Build history of the part. All positions in model axes, mm. A direction names the side the tool comes from. Round coordinates to 2 decimals unless told otherwise and drop trailing zeros. Write each loop counter-clockwise with the first axis right and the second up, starting at its lowest first coordinate (ties: lowest second). Pieces come first, ordered by that corner, then holes. Notation, with made-up numbers: M -21,48.25 L 4,48.25 A27 ccw 4,87.25 Z; hole C 77.25,80.25 d8. An arc over 180 degrees is marked long. Write item = value, one per line.
from build123d import *

# Parameters (mm, degrees)
BOSS_EXTRUDE1_DEPTH = 15
SKETCH2_R           = 2.1
CUT_EXTRUDE1_DEPTH  = 66.331515512
FILLET2_R           = 1.905


with BuildPart() as part:
    # Sketch1 → Boss-Extrude1 (new body)
    with BuildSketch(Plane(origin=(0, 0, 0), x_dir=(0, 0, -1), z_dir=(1, 0, 0))):
        with BuildLine():
            Line((-6.5, 0), (-10.31, 0))
            Line((-10.31, 0), (-10.31, 25.4))
            add(Edge.make_bspline(
                [(-10.31, 25.4), (-3.368064257, 40.422360056), (-3, 57.15)],
                knots=[0, 0, 0, 1, 1, 1], degree=2))
            ThreePointArc((-3, 57.15), (0, 60.15), (3, 57.15))
            add(Edge.make_bspline(
                [(10.31, 25.4), (3.368064257, 40.422360056), (3, 57.15)],
                knots=[0, 0, 0, 1, 1, 1], degree=2))
            Line((10.31, 25.4), (10.31, 0))
            Line((10.31, 0), (6.5, 0))
            Line((6.5, 0), (6.5, 25.4))
            Line((6.5, 25.4), (-6.5, 25.4))
            Line((-6.5, 25.4), (-6.5, 0))
        make_face()
    extrude(amount=BOSS_EXTRUDE1_DEPTH)

    # Sketch2 → Cut-Extrude1 (cut, through all)
    with BuildSketch(Plane(origin=(0, 0, -10.31), x_dir=(-1, 0, 0), z_dir=(0, 0, -1))):
        with Locations((-7.5, 7)):
            Circle(SKETCH2_R)
        with Locations((-7.5, 17)):
            Circle(SKETCH2_R)
    extrude(amount=-CUT_EXTRUDE1_DEPTH, mode=Mode.SUBTRACT)

    # Fillet2
    fillet2_edges = [part.edges().sort_by_distance(p)[0] for p in [
        (7.5, 25.4, -10.31),
        (7.5, 0, -10.31),
        (7.5, 0, -6.5),
        (7.5, 0, 6.5),
        (7.5, 0, 10.31),
        (7.5, 25.4, -6.5),
        (7.5, 25.4, 6.5),
        (7.5, 25.4, 10.31),
    ]]
    fillet(fillet2_edges, radius=FILLET2_R - 0.0001)  # a hair under: the kernel refuses the full size


solid = part.part
1. Band-saw the part on B-B (x = 7.5). Count the separate pieces of the cut face and the enclosed holes in it, plus the area to 3 significant figures.
Responses:
separate_pieces = 5
enclosed_holes = 0
area = 491 mm²
2. Mould opens along Y. For faces 3 (the face through (7.773, 9.082, -8.432)), 4 (the face through (7, 13, 6.5)), 5 (the face through (7.4, 60.15, 0.07)), 6 (the face through (7, 25.4, 0)) say: pulls with the +Y half, pulls with the -Y half, needs draft (parallel to the pull), parting line crosses it, or undercut.
Responses:
face_3 = undercut
face_4 = needs draft
face_5 = pulls with the +Y half
face_6 = pulls with the -Y half
3. Band-saw the part on A-A (y = 17). List the corners of the cut face in (x, z), plus the area to 3 significant figures.
Responses:
outline = M 0,-10.31 L 5.4,-10.31 L 5.4,-6.5 L 0,-6.5 Z; M 0,6.5 L 5.4,6.5 L 5.4,10.31 L 0,10.31 Z; M 9.6,-10.31 L 15,-10.31 L 15,-6.5 L 9.6,-6.5 Z; M 9.6,6.5 L 15,6.5 L 15,10.31 L 9.6,10.31 Z
area = 82.3 mm²
4. Flat gauge pins, fed straight in: pin 1 (1 mm diameter, centred on x = 4.5, y = 33, fed in from -Z); pin 2 (3 mm diameter, centred on x = 9.5, y = 34, fed in from +Z); pin 3 (7.5 mm diameter, centred on x = 9, z = 1.5, fed in from -Y). Where does each tip first touch, or does it go through?
Responses:
pin_1 = -7.43
pin_2 = 7.43
pin_3 = 25.28
5. Band-saw the part on C-C (z = 0). List the corners of the cut face in (x, y).
Responses:
outline = M 0,25.4 L 15,25.4 L 15,60.15 L 0,60.15 Z
6. Tool access for faces 1 (the face through (7.605, 24.827, 5.957)), 2 (the face through (7, 13, 10.31)): list every direction of +Z, -Z, +X, -X, +Y, -Y with a clear straight run to the whole face (end or side of a thin tool).
Responses:
face_1 = +X, -X, -Y
face_2 = +Z, +X, -X, +Y, -Y
7. Probe probe 1 along Z at (x, y) = (11, 18.5); probe 2 along X at (y, z) = (16, -9); probe 3 along Z at (x, y) = (8.75, 36.5). List the from-to ranges inside material, lowest first.
Responses:
probe_1 = -10.31 to -6.5, 6.5 to 10.31
probe_2 = 0 to 5.65, 9.35 to 15
probe_3 = -6.15 to 6.15
